CAD build for the part. Positions are in the model's coordinates, mm. A direction names the side the tool comes from. Give positions to 0.01 mm unless a question says otherwise; leave off trailing zeros. Loops run counter-clockwise (first coordinate to the right, second up) from the corner with the lowest first, then second, coordinate; pieces in that order, holes last. Notation, with made-up numbers: M 23.25,80 L 30.25,80 A14 cw 30.25,104 Z; hole C 48,10.25 d6. An arc over 180 degrees is marked long. One line per question, with ' | ' between items.
Autodesk Fusion 360 part; units mm, degrees
sketch "Sketch1" plane through (0, 0, 0) normal (0, 1, 0) x (1, 0, 0)
  line L0 (0, 0) -> (-12.5, 0)
  line L1 (-12.5, 0) -> (-12.5, -11.5)
  line L2 (-12.5, -11.5) -> (0, -11.5)
  line L3 (0, -11.5) -> (0, 0)
  dimension "d1" = 12.5
  dimension "d2" = 11.5
extrude "Extrude1" add sketch "Sketch1" along normal blind 2
sketch "Sketch2" plane through (0, 0, 0) normal (0, -1, 0) x (1, 0, 0)
  line L0 (0, 0) -> (0, 11.5)
  line L1 (0, 11.5) -> (-12.5, 11.5)
  line L2 (-12.5, 11.5) -> (-12.5, 0)
  line L3 (-12.5, 0) -> (0, 0)
  line L4 (0, 0) -> (-2.1, 0)
  line L5 (-2.1, 0) -> (-2.1, 11.5)
  line L6 (-2.1, 11.5) -> (0, 11.5)
  line L7 (0, 11.5) -> (0, 0)
  dimension "d5" = 2.1
extrude "Extrude2" add sketch "Sketch2" along normal blind 1 contours L0 L1 L3 L4 L5 L6 L7
sketch "Sketch3" plane through (0, 0, 0) normal (0, -1, 0) x (1, 0, 0)
  line L0 (-2.1, 0) -> (-2.1, 11.5)
  line L1 (-2.1, 11.5) -> (-12.5, 11.5)
  line L2 (-12.5, 11.5) -> (-12.5, 0)
  line L3 (-12.5, 0) -> (-2.1, 0)
  spline S0 degree 5 poles (0, 10) (0.1223, 10) (0.3487, 9.9879) (0.6334, 9.9337) (0.9192, 9.7757) (1.1918, 9.3796) (1.4459, 8.741) (1.6857, 7.8807) (1.8409, 6.9019) (1.9033, 5.8712) (1.8768, 4.8517) (1.7821, 3.8919) (1.6397, 3.0312) (1.4634, 2.2995) (1.248, 1.7174) (0.9635, 1.2964) (0.6503, 1.0932) (0.3517, 1.0169) (0.1223, 1) (0, 1) knots 0 0 0 0 0 0 0.066667 0.133333 0.2 0.266667 0.333333 0.4 0.466667 0.533333 0.6 0.666667 0.733333 0.8 0.866667 0.933333 1 1 1 1 1 1
  line L4 (0.2641, 6.4) -> (0.2641, 4.6)
  arc A0 (0.2641, 4.6) -> (1.344, 4.6) centre (0.804, 4.6) ccw
  line L5 (1.344, 4.6) -> (1.344, 6.4)
  arc A1 (1.344, 6.4) -> (0.2641, 6.4) centre (0.804, 6.4) ccw
  line L6 (0.804, 6.4) -> (0.804, 4.6) construction
  line L7 (1.2151, 9.4545) -> (1.7849, 7.5455)
  line L8 (0, 10) -> (0, 1)
  line L9 (-1, 10) -> (1, 10)
  line L10 (1, 1) -> (-1, 1)
  point P0 (1.5, 8.5)
  point P1 (1.5, 2.5)
  point P2 (0.804, 5.5)
  dimension "d8" = 5.5
  dimension "d9" = 1.8
extrude "Extrude3" add sketch "Sketch3" against normal blind 0.5 contours S0 L8
sketch "Sketch4" plane through (0, 0, 0) normal (0, -1, 0) x (1, 0, 0)
  line L0 (-2.1, 0) -> (-2.1, 11.5)
  line L1 (-2.1, 11.5) -> (-12.5, 11.5)
  line L2 (-12.5, 11.5) -> (-12.5, 0)
  line L3 (-12.5, 0) -> (-2.1, 0)
  line L4 (-11.5, 10.5) -> (-2.5, 10.5)
  line L5 (-2.5, 10.5) -> (-2.5, 8)
  line L6 (-2.5, 8) -> (-11.5, 8)
  line L7 (-11.5, 8) -> (-11.5, 10.5)
  line L8 (-2.5, 0.5) -> (-11.5, 0.5)
  line L9 (-11.5, 0.5) -> (-11.5, 3)
  line L10 (-11.5, 3) -> (-2.5, 3)
  line L11 (-2.5, 3) -> (-2.5, 0.5)
  line L12 (-11, 7.5) -> (-2.5, 7.5)
  line L13 (-2.5, 7.5) -> (-2.5, 6)
  line L14 (-2.5, 6) -> (-11, 6)
  line L15 (-11, 6) -> (-11, 7.5)
  line L16 (-2.5, 3.5) -> (-11, 3.5)
  line L17 (-11, 3.5) -> (-11, 5)
  line L18 (-11, 5) -> (-2.5, 5)
  line L19 (-2.5, 5) -> (-2.5, 3.5)
extrude "Extrude4" cut sketch "Sketch4" against normal blind 0.01 contours L4 L5 L6 L7 | L8 L9 L10 L11 | L12 L13 L14 L15 | L16 L17 L18 L19
Item 1: Saw through at B-B on y = 1.1. Give the cut face in (x, z).
Conclusion:
outline: M -12.5,0 L 0,0 L 0,11.5 L -12.5,11.5 Z
Item 2: Drill centre lines: line 1 along Y through (x, z) = (-2.75, 5.25); line 2 along X through (y, z) = (-0.25, 11); line 3 along X through (y, z) = (1.5, 7). Where is each one in solid material? Low to high. Write a range as [from, to].
Conclusion:
line 1: [0, 2] | line 2: [-2.1, 0] | line 3: [-12.5, 0]
Item 3: 3-axis set-ups, long thin cutter, end or side, ignore diameter. For faces 1 (the flat face through (1.6, 0.5, 5.6)), 2 (the flat face through (1.6, 0, 5.6)): which of +Z, -Z, +X, -X, +Y, -Y reach the whole face in a straight line?
Conclusion:
face 1: +Z, -Z, +X, +Y | face 2: +Z, -Z, +X, -Y
Item 4: Drop flat-ended pins along their axis: P1, Ø5, axis at x = -7.5, z = 3, coming from the -Y side; P2, Ø0.6, axis at x = 1, z = 6, coming from the +Y side. Give the stop position or say it passes through.
Conclusion:
P1: y = 0 | P2: through
